Build history of the part. All positions in model axes, mm. Give positions to 0.01 mm unless a question says otherwise; leave off trailing zeros. Order: outer loops, then holes, each group sorted by start corner. A loop starts at its lowest first (then second) coordinate and runs counter-clockwise, first axis right, second up. Notation, with made-up numbers: (82, 27.25) - (96, 27.25) arc R19 cw to (96, 37.25) - close; hole circle Ø5 at (77.25, -35.5). An arc over 180 degrees is marked (long way). Use a Markdown table: item, result. Add a question column.
(1) Slice it at A-A (x = 8). Write the cut outline in (y, z), then the cut area to 3 significant figures.
(2) Slice it at D-D (z = 5). Write the cut outline in (x, y).
(3) Slice it at B-B (x = 0). Write the cut outline in (y, z).
(4) Flat gauge pin, fed straight in: pin 1 (1 mm diameter, centred on x = 6, y = -0.5, fed in from -Z). Where does the tip first touch, or does it go through?
(5) Slice it at C-C (z = 19.5). Write the cut outline in (x, y).
(6) Wall check: line 1 (Z direction, x = 5.5, y = -0.55); line 2 (X direction, y = -0.95, z = 20.75); line 3 (Z direction, x = -8, y = -0.5). Give the ranges that are in metal, low to high.
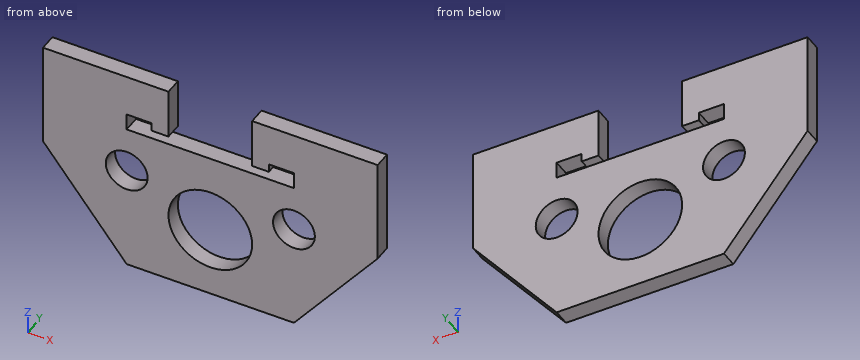
Solid Edge part; units mm, degrees
sketch "Sketch1" plane through (0, 0, 0) normal (0, -1, 0) x (1, 0, 0)
  line L0 (20, 12.5) -> (20, 25)
  line L1 (5, 25) -> (20, 25)
  line L2 (5.0015, 19) -> (5, 25)
  line L3 (7.0015, 19) -> (5.0015, 19)
  line L4 (7.0015, 20) -> (7.0015, 19)
  line L5 (10, 20) -> (7.0015, 20)
  line L6 (10, 18) -> (10, 20)
  line L7 (-10, 18) -> (10, 18)
  line L8 (-10, 20) -> (-10, 18)
  line L9 (-10, 20) -> (-7, 20)
  line L10 (-7, 20) -> (-7, 19)
  line L11 (-7, 19) -> (-5, 19)
  line L12 (-5, 19) -> (-5, 20)
  line L13 (-5, 25) -> (-5, 20)
  line L14 (-5, 25) -> (-20, 25)
  line L15 (-20, 25) -> (-20, 12.5)
  line L16 (-20, 12.5) -> (-10, 0)
  line L17 (-10, 0) -> (-10, 0) construction
  line L18 (-10, 0) -> (10, 0)
  line L19 (10, 0) -> (10, 0) construction
  line L20 (20, 12.5) -> (10, 0)
  circle A0 centre (0, 8.4952) radius 5
  circle A1 centre (10, 12.5) radius 2.5
  circle A2 centre (-10, 12.5) radius 2.5
extrude "ExtrudedProtrusion_1" add sketch "Sketch1" along normal blind 2
properties material "Acrylic, high impact grade"
Solution:
| question | item | result |
|---|---|---|
| 1 | outline | (-2, 0) - (0, 0) - (0, 11) - (-2, 11) - close; (-2, 14) - (0, 14) - (0, 18) - (-2, 18) - close; (-2, 20) - (0, 20) - (0, 25) - (-2, 25) - close |
| 1 | area | 40.0 mm2 |
| 2 | outline | (-14, -2) - (-3.58, -2) - (-3.58, 0) - (-14, 0) - close; (3.58, -2) - (14, -2) - (14, 0) - (3.58, 0) - close |
| 3 | outline | (-2, 0) - (0, 0) - (0, 3.5) - (-2, 3.5) - close; (-2, 13.5) - (0, 13.5) - (0, 18) - (-2, 18) - close |
| 4 | pin 1 | z = 0 |
| 5 | outline | (-20, -2) - (-10, -2) - (-10, 0) - (-20, 0) - close; (-7, -2) - (-5, -2) - (-5, 0) - (-7, 0) - close; (5, -2) - (7, -2) - (7, 0) - (5, 0) - close; (10, -2) - (20, -2) - (20, 0) - (10, 0) - close |
| 6 | line 1 | 0 to 18, 19 to 25 |
| 6 | line 2 | -20 to -5, 5 to 20 |
| 6 | line 3 | 0 to 11, 14 to 18, 20 to 25 |
